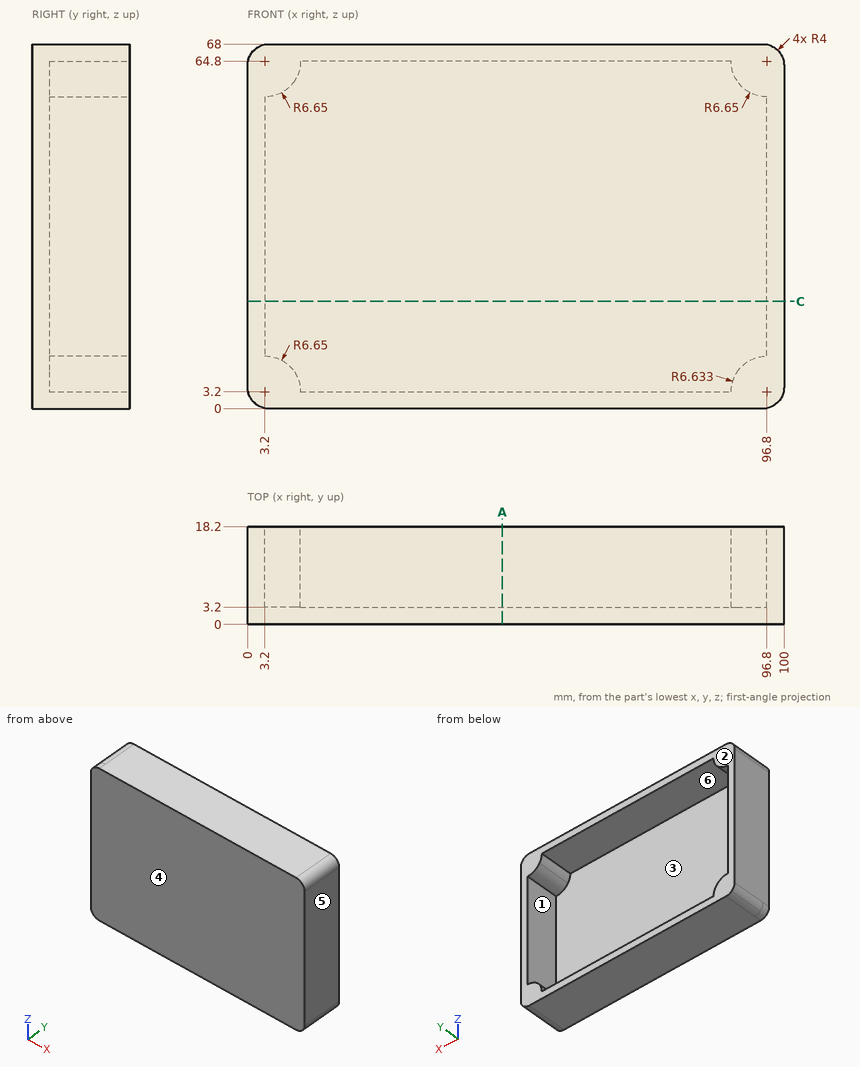
Geometry check sheet. Reference: drawing and pictorial views, mm from the part's lowest x, y, z. A direction names the side the tool comes from. Give positions to 0.01 mm unless a question says otherwise; leave off trailing zeros. Order: outer loops, then holes, each group sorted by start corner. A loop starts at its lowest first (then second) coordinate and runs counter-clockwise, first axis right, second up. Notation, with made-up numbers: M -27.75,-10 L -11.75,-10 A15 ccw -11.75,6 Z; hole C 28,71.25 d11. An arc over 180 degrees is marked long. Use one line per item in the form item = value. Start each with the question number.
Q1. Go/stop test with a flat-tipped pin: pin 1 Ø6 at (x, y) = (64, 2) entering from -Z. Record where the tip stops, or that it passes through.
Q2. Mould release check, pull along X, two halves, no side actions. Record for the marked faces 3, 4, 5 and 6: +X half, -X half, draft (parallel to the pull), parting line (faces both ways), or undercut.
Q3. Scan lines: line 1 along Z through (x, y) = (40, 17); line 2 along X through (y, z) = (9.5, 16); line 3 along Y through (x, z) = (44, 9.5). Record each from-to range of solid material in increasing order. Write a range as [from, to].
Q4. Section check A-A (x = 47.5). Enter the section's corners in (y, z), then the cut area to 3 significant figures.
Q5. Section check C-C (z = 20). Enter the section's corners in (x, y), then the cut area to 3 significant figures.
Q6. Access from +Z, -Z, +X, -X, +Y, -Y to the whole of each face (thin tool, end or side, straight path). Record for the marked faces 1 and 2.
Evaluation:
q1.pin_1 = 0
q2.face_3 = undercut
q2.face_4 = draft
q2.face_5 = +X half
q2.face_6 = undercut
q3.line_1 = [0, 3.2], [64.8, 68]
q3.line_2 = [0, 3.2], [96.8, 100]
q3.line_3 = [0, 3.2]
q4.outline = M 0,0 L 18.2,0 L 18.2,3.2 L 3.2,3.2 L 3.2,64.8 L 18.2,64.8 L 18.2,68 L 0,68 Z
q4.area = 314 mm2
q5.outline = M 0,0 L 100,0 L 100,18.2 L 96.8,18.2 L 96.8,3.2 L 3.2,3.2 L 3.2,18.2 L 0,18.2 Z
q5.area = 416 mm2
q6.face_1 = +Y
q6.face_2 = +Z, -Z, +X, -X, +Y
